Check sheet for the drawn part. Datum: minimum x, y, z corner. Units: mm. A direction names the side the tool comes from. Coordinates: 2 decimals unless noted, no trailing zeros. Order: outer loops, then holes, each group sorted by start corner. A loop starts at its lowest first (then second) coordinate and runs counter-clockwise, first axis right, second up. Notation, with made-up numbers: M 62.5,54.25 L 69.5,54.25 A29 ccw 69.5,87.25 Z; hole C 20,87 d9. An arc over 180 degrees is marked long. Return JSON: item names as keys, results as strings. Group by question number.
Q1. Thickness scan on probe 1 along Y at (x, z) = (1.6, 3.05); probe 2 along Y at (x, z) = (3.85, 3.3); probe 3 along Z at (x, y) = (2.95, 3.7) (1 decimal). Record the ranges inside material, lowest first.
Q2. Section check C-C, the plane z = 2.85. Enter the section's corners in (x, y), then the cut area to 3 significant figures.
Q3. Go/stop test with a flat-tipped pin: pin 1 Ø0.6 at (x, z) = (2, 2) entering from +Y. Record where the tip stops, or that it passes through.
Q4. Section check A-A, the plane x = 2.25. Enter the section's corners in (y, z).
Q5. Mould release check, pull along Z, two halves, no side actions. Record for the marked faces 1, 2 and 3: pulls with the +Z half, pulls with the -Z half, needs draft (parallel to the pull), parting line crosses it, or undercut.
Q6. Section check B-B, the plane y = 1.45. Enter the section's corners in (x, z).
Q7. Access from +Z, -Z, +X, -X, +Y, -Y to the whole of each face (thin tool, end or side, straight path). Record for the marked faces 4, 5 and 6.
Q8. Section check D-D, the plane z = 3.35. Enter the section's corners in (x, y).
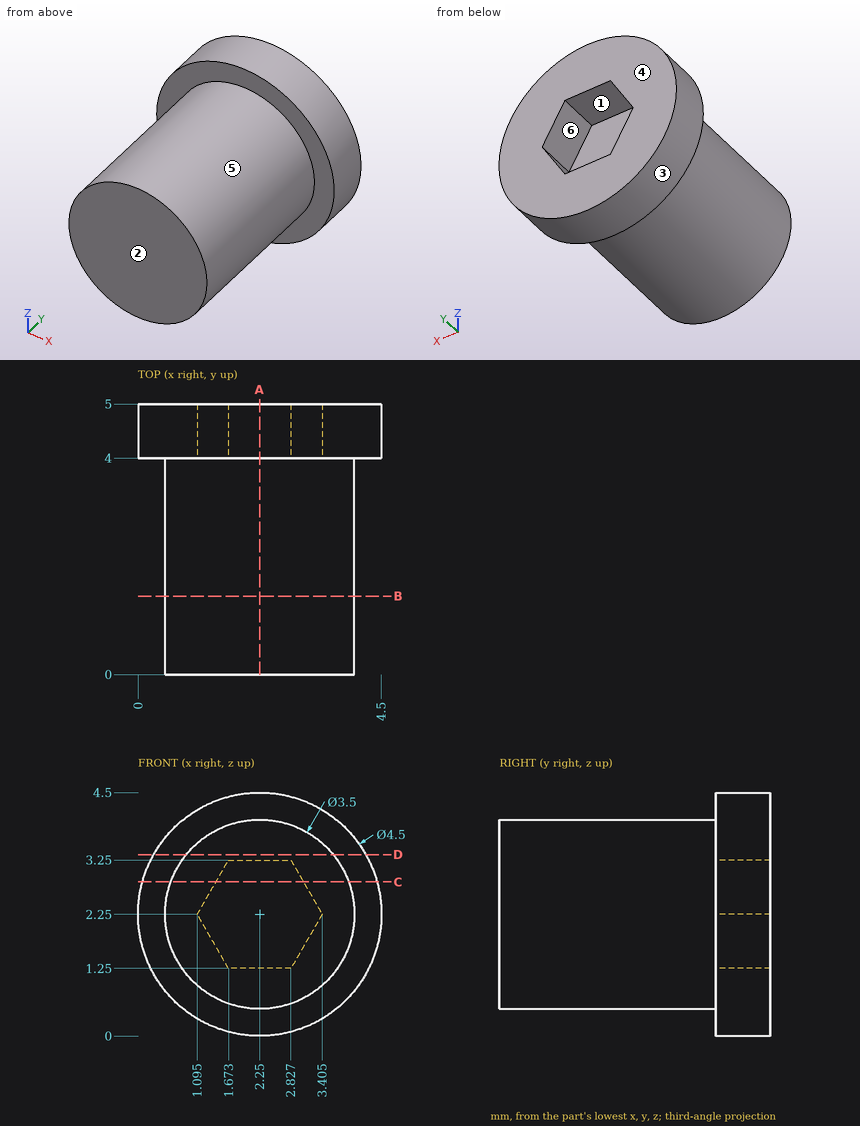
Numbers:
{
 "1": {"probe 1": "y = 0 to 4", "probe 2": "y = 4 to 5", "probe 3": "z = 0.6 to 3.9"},
 "2": {"outline": "M 0.08,4 L 0.61,4 L 0.61,0 L 3.89,0 L 3.89,4 L 4.42,4 L 4.42,5 L 3.06,5 L 3.06,4 L 1.44,4 L 1.44,5 L 0.08,5 Z", "area": "15.9 mm2"},
 "3": {"pin 1": "stops at y = 4"},
 "4": {"outline": "M 0,0.5 L 4,0.5 L 4,0 L 5,0 L 5,1.25 L 4,1.25 L 4,3.25 L 5,3.25 L 5,4.5 L 4,4.5 L 4,4 L 0,4 Z"},
 "5": {"face 1": "undercut", "face 2": "needs draft", "face 3": "parting line crosses it"},
 "6": {"outline": "C 2.25,2.25 d3.5"},
 "7": {"face 4": "+Z, -Z, +X, -X, +Y", "face 5": "-Y", "face 6": "+Y"},
 "8": {"outline": "M 0.29,4 L 0.89,4 L 0.89,0 L 3.61,0 L 3.61,4 L 4.21,4 L 4.21,5 L 0.29,5 Z"}
}
